from build123d import *

# Parameters (mm, degrees)
SKETCH019_R            = 2.5
PAD013_DEPTH           = 8
POCKET_DEPTH           = 4.5
LINEARPATTERN001_COUNT = 2
LINEARPATTERN001_PITCH = 38


with BuildPart() as linearpattern001:
    # Sketch019 → Pad013 (new body)
    with BuildSketch(Plane.XY.offset(8)):
        Polygon((8, 192), (32, 150.430781), (32, -192), (8, -192), align=None)
        with Locations((20, -115)):
            Circle(SKETCH019_R, mode=Mode.SUBTRACT)
        with Locations((20, -153)):
            Circle(SKETCH019_R, mode=Mode.SUBTRACT)
    extrude(amount=PAD013_DEPTH)

    # Sketch021 → Pocket (cut)
    with BuildSketch(Plane(origin=(0, 0, 8), x_dir=(1, 0, 0), z_dir=(0, 0, -1))):
        Polygon((20, 123), (13.071797, 111), (26.928203, 111), align=None)
    pocket = extrude(amount=-POCKET_DEPTH, mode=Mode.SUBTRACT)

    # LinearPattern001: Pocket ×2
    with Locations(*[(0, -i * LINEARPATTERN001_PITCH, 0) for i in range(1, LINEARPATTERN001_COUNT)]):
        add(pocket, mode=Mode.SUBTRACT)


with BuildPart() as part_mirroring003:
    # Part__Mirroring003: instance of LinearPattern001
    add(linearpattern001.part.mirror(Plane(origin=(0, 0, 200), x_dir=(0, 1, 0), z_dir=(0, 0, 1))))


solid = part_mirroring003.part
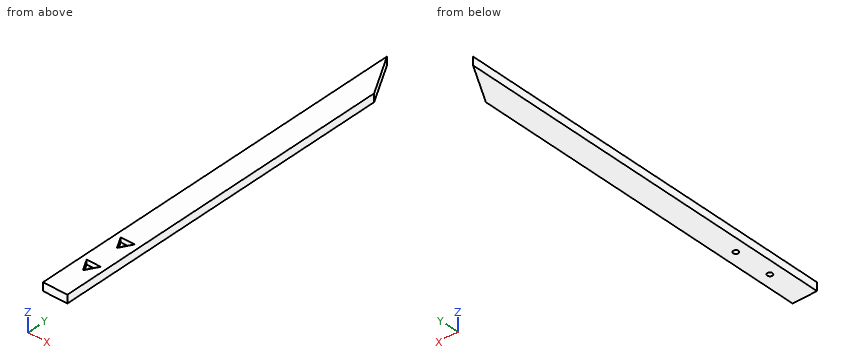
CAD build for the part. Positions are in the model's coordinates, mm. Round coordinates to 2 decimals unless told otherwise and drop trailing zeros. Loops run counter-clockwise (first coordinate to the right, second up) from the corner with the lowest first, then second, coordinate; pieces in that order, holes last.
(1) Cut at B-B (y = 167). Give the cut face in (x, z).
(2) Wall check: line 1 along Y through (x, z) = (20, 385.35); line 2 along X through (y, z) = (-115, 384.85); line 3 along Y through (x, z) = (23, 391.5). Give the ranges that are in metal, low to high.
(3) Drop a flat-ended pin along its axis: pin 1 (1.5 mm diameter, centred on x = 18.5, z = 386.5, fed in from +Y). Give the stop position or say it passes through.
(4) Cut at A-A (z = 390.25). Give the cut face in (x, y), plus the area to 3 significant figures.
Findings below:
1. outline: (8, 384) - (22.43, 384) - (22.43, 392) - (8, 392) - close
2. line 1: y = -192 to -155.5, -150.5 to -117.5, -112.5 to 171.22
2. line 2: x = 8 to 17.5, 22.5 to 32
2. line 3: y = -192 to -155.8, -149 to -117.8, -111 to 166.02
3. pin 1: stops at y = 175.11
4. outline: (8, -192) - (32, -192) - (32, 150.43) - (8, 192) - close; hole (13.07, -149) - (20, -161) - (26.93, -149) - close; hole (13.07, -111) - (20, -123) - (26.93, -111) - close
4. area: 8,550 mm2
